Here's the drawing with two shaded views (mm, measured from the low corner). I have some questions. Round coordinates to 2 decimals unless told otherwise and drop trailing zeros. Order: outer loops, then holes, each group sorted by start corner. A loop starts at its lowest first (then second) coordinate and runs counter-clockwise, first axis right, second up. Notation, with made-up numbers: (-15, 1.25) - (26, 1.25) arc R14 cw to (26, 11.25) - close; hole circle Ø7 at (74.25, 65.25). An arc over 180 degrees is marked (long way). Return JSON: item names as keys, results as strings. Group by question number.
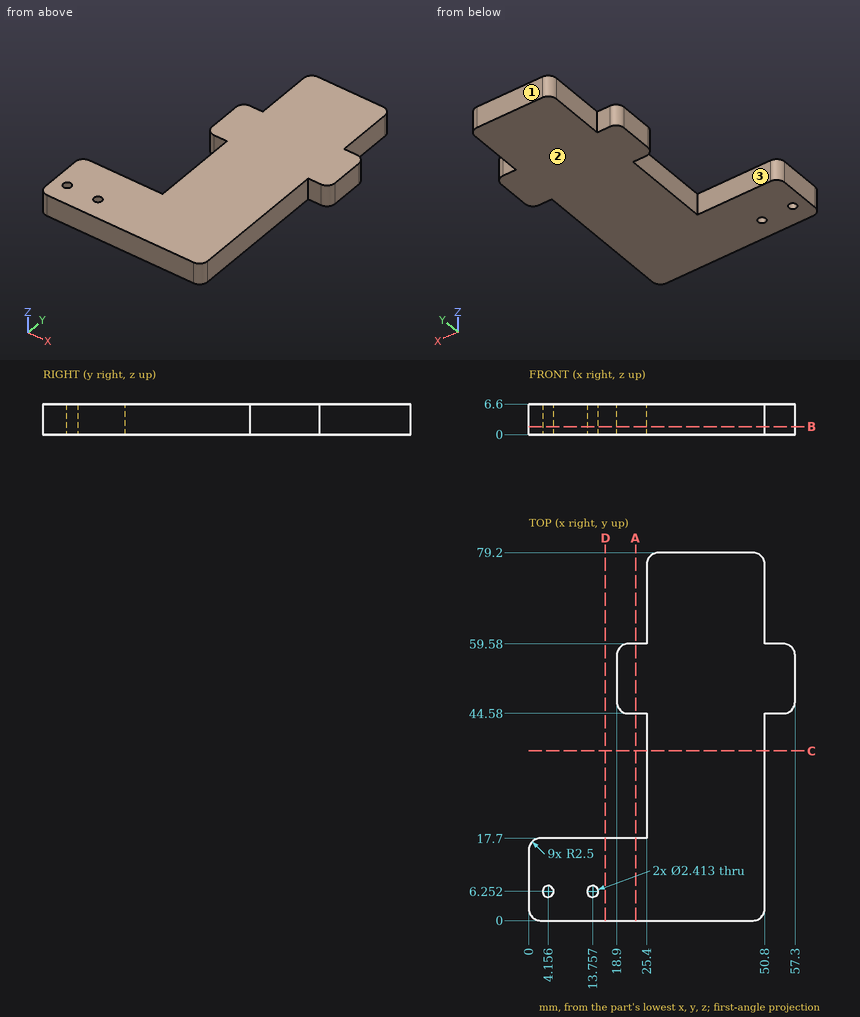
1) We'd pull the mould along Y, two halves only. Please class the marked faces 1, 2 and 3: +Y half, -Y half, draft (parallel to the pull), parting line (faces both ways), or undercut.
2) Will these pins go through, and if not, where does the flat tip stop? pin 1 (2 mm diameter, centred on x = 53, z = 3.5, fed in from -Y); pin 2 (2 mm diameter, centred on y = 65.5, z = 1.5, fed in from +X); pin 3 (3 mm diameter, centred on y = 25.5, z = 1, fed in from -X).
3) I want a section at A-A, the plane x = 23. List the corners of the cut face in (y, z) for me.
4) If I drill on line 1 along X through (y, z) = (65.5, 1); line 2 along X through (y, z) = (5.5, 4.25) (1 decimal); line 3 along Y through (x, z) = (21, 1.5), over which ranges is the centre line in solid material (lowest first)? Write a range as from..to.
5) I want a section at D-D, the plane x = 16.5. List the corners of the cut face in (y, z) for me, plus the area to 3 significant figures.
6) I want a section at B-B, the plane z = 1.75. List the corners of the cut face in (x, y) for me.
7) I want a section at C-C, the plane y = 36.5. List the corners of the cut face in (x, z) for me, plus the area to 3 significant figures.
Outcome:
{
 "1": {"face 1": "+Y half", "face 2": "draft", "face 3": "undercut"},
 "2": {"pin 1": "y = 44.58", "pin 2": "x = 50.8", "pin 3": "x = 25.4"},
 "3": {"outline": "(0, 0) - (17.7, 0) - (17.7, 6.6) - (0, 6.6) - close; (44.58, 0) - (59.58, 0) - (59.58, 6.6) - (44.58, 6.6) - close"},
 "4": {"line 1": "25.4..50.8", "line 2": "0..3.2, 5.1..12.8, 14.7..50.8", "line 3": "0..17.7, 44.61..59.55"},
 "5": {"outline": "(0, 0) - (17.7, 0) - (17.7, 6.6) - (0, 6.6) - close", "area": "117 mm^2"},
 "6": {"outline": "(0, 2.5) arc R2.5 ccw to (2.5, 0) - (48.3, 0) arc R2.5 ccw to (50.8, 2.5) - (50.8, 44.58) - (54.8, 44.58) arc R2.5 ccw to (57.3, 47.08) - (57.3, 57.08) arc R2.5 ccw to (54.8, 59.58) - (50.8, 59.58) - (50.8, 76.7) arc R2.5 ccw to (48.3, 79.2) - (27.9, 79.2) arc R2.5 ccw to (25.4, 76.7) - (25.4, 59.58) - (21.4, 59.58) arc R2.5 ccw to (18.9, 57.08) - (18.9, 47.08) arc R2.5 ccw to (21.4, 44.58) - (25.4, 44.58) - (25.4, 17.7) - (2.5, 17.7) arc R2.5 ccw to (0, 15.2) - close; hole circle Ø2.41 at (4.16, 6.25); hole circle Ø2.41 at (13.76, 6.25)"},
 "7": {"outline": "(25.4, 0) - (50.8, 0) - (50.8, 6.6) - (25.4, 6.6) - close", "area": "168 mm^2"}
}
